from build123d import *

# Parameters (mm, degrees)
SKETCH_1_R               = 8.5
SKETCH_1_R_2             = 3.6
SKETCH_1_R_3             = 1.25
SKETCH_1_R_4             = 0.6
EXTRUDE_1_DEPTH          = 9
SKETCH_2_R               = 4.3
CUT_EXTRUDE_1_DEPTH      = 0.8
SKETCH_3_R               = 5.9
SKETCH_3_R_2             = 3.6
EXTRUDE_2_DEPTH          = 2.5
SKETCH_5_R               = 4.3
CUT_EXTRUDE_2_DEPTH      = 0.8
EXTRUDE_3_DEPTH          = 7
CUT_EXTRUDE_6_DEPTH      = 1
CUT_EXTRUDE_6_DEPTH_BACK = 17
EXTRUDE_4_DEPTH          = 3.6
SKETCH_8_R               = 3.2
CUT_EXTRUDE_3_DEPTH      = 2


with BuildPart() as part:
    # 스케치1 → 보스-돌출1 (new body)
    with BuildSketch(Plane.XY):
        Circle(SKETCH_1_R)
        Circle(SKETCH_1_R_2, mode=Mode.SUBTRACT)
        with Locations((6.125, 0)):
            Circle(SKETCH_1_R_3, mode=Mode.SUBTRACT)
        with Locations((-6.8, 0)):
            Circle(SKETCH_1_R_4, mode=Mode.SUBTRACT)
    extrude(amount=EXTRUDE_1_DEPTH)

    # 스케치2 → 컷-돌출1 (cut)
    with BuildSketch(Plane.XY.offset(9)):
        Circle(SKETCH_2_R)
    extrude(amount=-CUT_EXTRUDE_1_DEPTH, mode=Mode.SUBTRACT)

    # 스케치3 → 보스-돌출2 (add)
    with BuildSketch(Plane(origin=(0, 0, 0), x_dir=(-1, 0, 0), z_dir=(0, 0, -1))):
        Circle(SKETCH_3_R)
        Circle(SKETCH_3_R_2, mode=Mode.SUBTRACT)
    extrude(amount=EXTRUDE_2_DEPTH)

    # 스케치4 → 컷-회전1 (revolve, cut)
    with BuildSketch(Plane(origin=(0, 0, 0), x_dir=(0, 0, -1), z_dir=(1, 0, 0))):
        Polygon((2.5, 5.9), (0, 5.9), (1.25, 4.6), align=None)
    revolve(axis=Axis((0, 0, 0), (0, 0, -1)), mode=Mode.SUBTRACT)

    # 스케치5 → 컷-돌출2 (cut)
    with BuildSketch(Plane(origin=(0, 0, -2.5), x_dir=(-1, 0, 0), z_dir=(0, 0, -1))):
        Circle(SKETCH_5_R)
    extrude(amount=-CUT_EXTRUDE_2_DEPTH, mode=Mode.SUBTRACT)

    # 스케치6 → 보스-돌출3 (add)
    with BuildSketch(Plane(origin=(0, 0, 0), x_dir=(-1, 0, 0), z_dir=(0, 0, -1))):
        with BuildLine():
            Line((-2.907171218, 7.987387277), (-2.359938989, 6.483879083))
            ThreePointArc((-2.359938989, 6.483879083), (0, 6.9), (2.359938989, 6.483879083))
            Line((2.359938989, 6.483879083), (2.907171218, 7.987387277))
            ThreePointArc((2.907171218, 7.987387277), (0, 8.5), (-2.907171218, 7.987387277))
        make_face()
    extrude(amount=EXTRUDE_3_DEPTH)

    # 스케치10 → 컷-돌출6 (cut, two sides)
    with BuildSketch(Plane(origin=(0, 0, -7), x_dir=(-1, 0, 0), z_dir=(0, 0, -1))) as cut_extrude_6_sk:
        with BuildLine():
            ThreePointArc((-2.907171218, 7.987387277), (0, -8.5), (2.907171218, 7.987387277))
            Line((2.907171218, 7.987387277), (2.359938989, 6.483879083))
            ThreePointArc((2.359938989, 6.483879083), (0, 6.9), (-2.359938989, 6.483879083))
            Line((-2.359938989, 6.483879083), (-2.907171218, 7.987387277))
        make_face()
    extrude(amount=CUT_EXTRUDE_6_DEPTH, mode=Mode.SUBTRACT)
    extrude(cut_extrude_6_sk.sketch, amount=-CUT_EXTRUDE_6_DEPTH_BACK, mode=Mode.SUBTRACT)

    # 스케치7 → 보스-돌출4 (add)
    with BuildSketch(Plane(origin=(0, 0, -7), x_dir=(-1, 0, 0), z_dir=(0, 0, -1))):
        with BuildLine():
            Line((-2.359938989, 6.483879083), (-2.359938989, 4.408025405))
            ThreePointArc((-2.359938989, 4.408025405), (0, -5), (2.359938989, 4.408025405))
            Line((2.359938989, 4.408025405), (2.359938989, 6.483879083))
            Line((2.359938989, 6.483879083), (2.907171218, 7.987387277))
            ThreePointArc((2.907171218, 7.987387277), (0, 8.5), (-2.907171218, 7.987387277))
            Line((-2.907171218, 7.987387277), (-2.359938989, 6.483879083))
        make_face()
    extrude(amount=EXTRUDE_4_DEPTH)

    # 스케치8 → 컷-돌출3 (cut)
    with BuildSketch(Plane(origin=(0, 0, -10.6), x_dir=(-1, 0, 0), z_dir=(0, 0, -1))):
        Circle(SKETCH_8_R)
    extrude(amount=-CUT_EXTRUDE_3_DEPTH, mode=Mode.SUBTRACT)


solid = part.part
For this review, take the finished solid that the model builds, in its own axes (mm). A direction names the side the tool comes from. Give positions to 0.01 mm unless a question says otherwise; leave off trailing zeros. Order: outer loops, then holes, each group sorted by start corner. A loop starts at its lowest first (then second) coordinate and runs counter-clockwise, first axis right, second up. Notation, with made-up numbers: (86, 22) -> (128, 22) arc R26 ccw to (128, 39) -> close; hole circle Ø8 at (-12.5, 45). An arc over 180 degrees is marked (long way). Write item = value, one per line.
1) Insertion check: pin 1 (4 mm diameter, centred on x = 2, y = 3, fed in from +Z); pin 2 (0.6 mm diameter, centred on y = 6, z = -9, fed in from +X); pin 3 (8 mm diameter, centred on y = 6, z = 3.5, fed in from +X). Each pin has a flat end and moves straight along its axis. Give the tip position at first contact, or say it passes through.
Findings:
pin_1 = -7
pin_2 = 2.36
pin_3 = 2.91
2) We need section B-B, the plane x = 0. Give the boundary of the cut face in (y, z), and give its area (3 significant figures).
Findings:
outline = (-5, -10.6) -> (-3.2, -10.6) -> (-3.2, -8.6) -> (3.2, -8.6) -> (3.2, -10.6) -> (8.5, -10.6) -> (8.5, 9) -> (6.9, 9) -> (6.9, -7) -> (-5, -7) -> close
area = 61.4 mm^2
3) We need section D-D, the plane y = 1.5. Give the boundary of the cut face in (x, z).
Findings:
outline = (-4.77, -10.6) -> (-2.83, -10.6) -> (-2.83, -8.6) -> (2.83, -8.6) -> (2.83, -10.6) -> (4.77, -10.6) -> (4.77, -7) -> (-4.77, -7) -> close
4) To check wall thickness, follow L1, parallel to Y at x = 0, z = -9.85; L2, parallel to Z at x = 0, y = 6; L3, parallel to Z at x = 0, y = 0. State the ranges of each line that lie inside material, in increasing order. Write a range as from..to.
Findings:
L1 = -5..-3.2, 3.2..8.5
L2 = -10.6..-7
L3 = -8.6..-7
5) For faces 4 (the face through (2.64, 7.25, -0.66)), 5 (the face through (0, 0, -8.6)), 6 (the face through (-2.36, 5, -9)), list the 3-axis set-ups (+Z, -Z, +X, -X, +Y, -Y) from which the entire face can be reached by the end or side of a thin tool; tool diameter is ignored.
Findings:
face_4 = +Z, -Z, +X
face_5 = -Z
face_6 = +Z, -Z, -X
6) We need section C-C, the plane z = -6. Give the boundary of the cut face in (x, y), and give its area (3 significant figures).
Findings:
outline = (-2.91, 7.99) -> (-2.36, 6.48) arc R6.9 cw to (2.36, 6.48) -> (2.91, 7.99) arc R8.5 ccw to start
area = 8.60 mm^2
7) We need section A-A, the plane y = 0. Give the boundary of the cut face in (x, z), and give its area (3 significant figures).
Findings:
outline = (-5, -10.6) -> (-3.2, -10.6) -> (-3.2, -8.6) -> (3.2, -8.6) -> (3.2, -10.6) -> (5, -10.6) -> (5, -7) -> (-5, -7) -> close
area = 23.2 mm^2
8) Draft analysis for pull direction X (two halves, no side actions). For faces 1 (the face through (2.36, 5, -9)), 2 (the face through (0, 6.9, 1.1)), 3 (the face through (0, 8.5, -0.7)), state which applies: pulls with the +X half, pulls with the -X half, needs draft (parallel to the pull), parting line crosses it, or undercut.
Findings:
face_1 = pulls with the +X half
face_2 = undercut
face_3 = parting line crosses it
